Autodesk Inventor part; units mm, degrees
ref_plane "YZ Plane" through (0, 0, 0) normal (1, 0, 0) x (0, 1, 0)
ref_plane "XZ Plane" through (0, 0, 0) normal (0, 1, 0) x (-1, 0, 0)
ref_plane "XY Plane" through (0, 0, 0) normal (0, 0, 1) x (1, 0, 0)
sketch "Sketch1" plane through (0, 0, 0) normal (1, 0, 0) x (0, 1, 0)
  line L0 (9.85, 22.75) -> (-9.85, 22.75)
  line L1 (-9.85, 22.75) -> (-9.85, -22.75)
  line L2 (-9.85, -22.75) -> (9.85, -22.75)
  line L3 (9.85, -22.75) -> (9.85, 22.75)
  circle A0 centre (0, 12.5) radius 8.5
  circle A1 centre (0, -12.5) radius 8.5
  line L4 (0, -12.5) -> (0, 12.5) construction
  point P0 (0, 0)
  point P1 (0, 0)
  point P2 (9.85, 0)
  point P3 (0, -22.75)
  dimension "d0" = 45.5
  dimension "d1" = 17
  dimension "d3" = 42
  dimension "d4" = 19.7
extrude "Extrusion1" add sketch "Sketch1" against normal blind 3.5 contours L3 L2 L1 L0 | A0 | A1
extrude "Extrusion2" add sketch "Sketch1" along normal blind 11.5 contours A0 | A1
properties part number "ultrasonic"
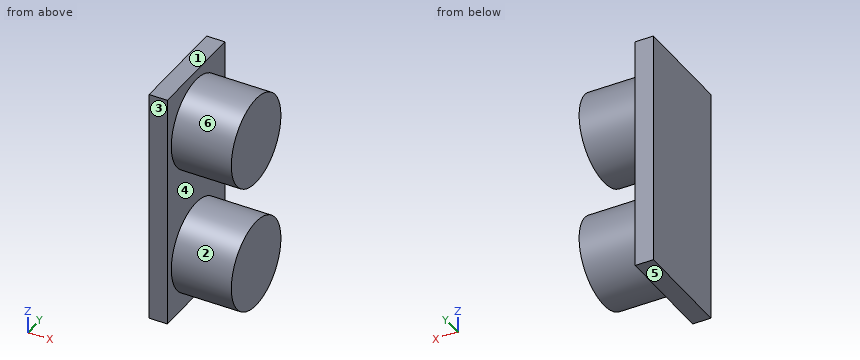
For this review, take the finished solid that the model builds, in its own axes (mm). Face numbers are marked on the shaded views. A direction names the side the tool comes from. Give positions to 0.01 mm unless a question says otherwise; leave off trailing zeros. Order: outer loops, then holes, each group sorted by start corner. A loop starts at its lowest first (then second) coordinate and runs counter-clockwise, first axis right, second up. Notation, with made-up numbers: (86, -4.75) -> (93, -4.75) arc R17 cw to (93, 23.25) -> close; hole circle Ø3 at (75, 41). An arc over 180 degrees is marked (long way). Write item = value, one per line.
1) To check wall thickness, follow L1, parallel to X at y = 3.25, z = -20.5; L2, parallel to Z at x = 1.75, y = -1.25; L3, parallel to Z at x = 2.5, y = -6.25. State the ranges of each line that lie inside material, in increasing order. Write a range as from..to.
Findings:
L1 = -3.5..0
L2 = -20.91..-4.09, 4.09..20.91
L3 = -18.26..-6.74, 6.74..18.26
2) We need section C-C, the plane x = 10.75. Give the boundary of the cut face in (y, z).
Findings:
outline = circle Ø17 at (0, -12.5); circle Ø17 at (0, 12.5)
3) We need section A-A, the plane z = -8.5. Give the boundary of the cut face in (x, y), and give its area (3 significant figures).
Findings:
outline = (-3.5, -9.85) -> (0, -9.85) -> (0, -7.5) -> (11.5, -7.5) -> (11.5, 7.5) -> (0, 7.5) -> (0, 9.85) -> (-3.5, 9.85) -> close
area = 241 mm^2
4) We need section D-D, the plane z = 19.5. Give the boundary of the cut face in (x, y).
Findings:
outline = (-3.5, -9.85) -> (0, -9.85) -> (0, -4.82) -> (11.5, -4.82) -> (11.5, 4.82) -> (0, 4.82) -> (0, 9.85) -> (-3.5, 9.85) -> close
5) Draft analysis for pull direction Z (two halves, no side actions). For the marked faces 1, 2, 3 and 4, state which applies: pulls with the +Z half, pulls with the -Z half, needs draft (parallel to the pull), parting line crosses it, or undercut.
Findings:
face_1 = pulls with the +Z half
face_2 = undercut
face_3 = needs draft
face_4 = undercut
6) We need section B-B, the plane y = 0. Give the boundary of the cut face in (x, z).
Findings:
outline = (-3.5, -22.75) -> (0, -22.75) -> (0, -21) -> (11.5, -21) -> (11.5, -4) -> (0, -4) -> (0, 4) -> (11.5, 4) -> (11.5, 21) -> (0, 21) -> (0, 22.75) -> (-3.5, 22.75) -> close
7) For the marked faces 5 and 6, list the 3-axis set-ups (+Z, -Z, +X, -X, +Y, -Y) from which the entire face can be reached by the end or side of a thin tool; tool diameter is ignored.
Findings:
face_5 = -Z, +X, -X, +Y, -Y
face_6 = +X
8) Insertion check: pin 1 (3 mm diameter, centred on x = 0.5, y = -4, fed in from +Z); pin 2 (8 mm diameter, centred on x = 6, z = -13.5, fed in from +Y); pin 3 (1.5 mm diameter, centred on x = 6, z = 1.5, fed in from -Y); pin 4 (1 mm diameter, centred on x = 2, z = 7, fed in from -Y). Each pin has a flat end and moves straight along its axis. Give the tip position at first contact, or say it passes through.
Findings:
pin_1 = 22.75
pin_2 = 8.5
pin_3 = through
pin_4 = -6.87
